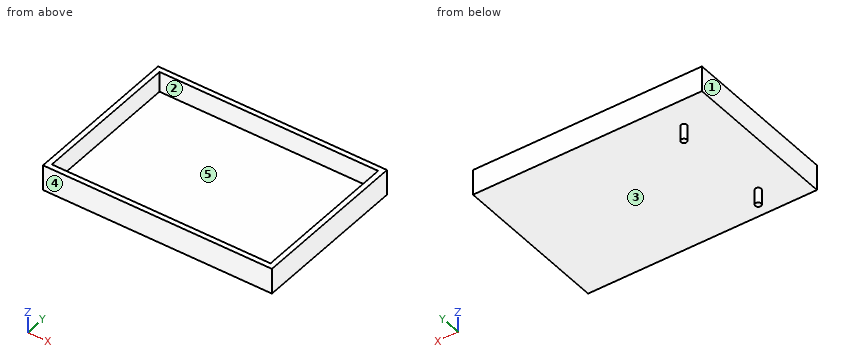
Autodesk Fusion 360 part; units mm, degrees
sketch "Sketch1" plane through (0, 0, 0) normal (0, 0, 1) x (1, 0, 0)
  line L0 (0, 0) -> (85.5, 0)
  line L1 (85.5, 0) -> (85.5, 58)
  line L2 (85.5, 58) -> (0, 58)
  line L3 (0, 58) -> (0, 0)
  line L4 (87.5, -2) -> (87.5, 60)
  line L5 (87.5, 60) -> (-2, 60)
  line L6 (-2, 60) -> (-2, -2)
  line L7 (-2, -2) -> (87.5, -2)
  dimension "d1" = 85.5
  dimension "d2" = 58
  dimension "d3" = 2
extrude "Extrude1" add sketch "Sketch1" along normal blind 10
sketch "Sketch2" plane through (0, 0, 0) normal (0, 0, 1) x (1, 0, 0)
  line L0 (0, 0) -> (85.5, 0)
  line L1 (85.5, 0) -> (85.5, 58)
  line L2 (85.5, 58) -> (0, 58)
  line L3 (0, 58) -> (0, 0)
  point P0 (85.5, 58)
extrude "Extrude2" add sketch "Sketch2" along normal blind 2
sketch "Sketch3" plane through (0, 0, 0) normal (0, 0, -1) x (1, 0, 0)
  line L0 (87.5, 2) -> (-2, 2)
  line L1 (-2, 2) -> (-2, -60)
  line L2 (-2, -60) -> (87.5, -60)
  line L3 (87.5, -60) -> (87.5, 2)
  line L4 (-2, -29) -> (87.5, -29)
  circle A0 centre (13, -9) radius 1.125
  circle A1 centre (13, -49) radius 1.125
  dimension "d8" = 2.25
  dimension "d9" = 2.25
  dimension "d10" = 20
  dimension "d11" = 20
  dimension "d14" = 15
extrude "Extrude3" add sketch "Sketch3" along normal blind 6 contours A0 | A1
sketch "Sketch4" plane through (0, 0, 0) normal (0, 0, -1) x (1, 0, 0)
  circle A0 centre (13, -9) radius 1.125
  circle A1 centre (13, -49) radius 1.125
  line L0 (87.5, 2) -> (-2, 2)
  line L1 (-2, 2) -> (-2, -60)
  line L2 (-2, -60) -> (87.5, -60)
  line L3 (87.5, -60) -> (87.5, 2)
For this review, take the finished solid that the model builds, in its own axes (mm). Face numbers are marked on the shaded views. A direction names the side the tool comes from. Round coordinates to 2 decimals unless told otherwise and drop trailing zeros. Order: outer loops, then holes, each group sorted by start corner. A loop starts at its lowest first (then second) coordinate and runs counter-clockwise, first axis right, second up.
Q1. We need section C-C, the plane y = 9. Give the boundary of the cut face in (x, z) (3 decimals).
Findings below:
outline: (-2, 0) - (11.875, 0) - (11.875, -6) - (14.125, -6) - (14.125, 0) - (87.5, 0) - (87.5, 10) - (85.5, 10) - (85.5, 2) - (0, 2) - (0, 10) - (-2, 10) - close
Q2. Machinability: for the marked faces 4 and 5, which of the approach directions +Z, -Z, +X, -X, +Y, -Y give a long, thin tool a straight path to every point of the face, cutting with its end or side? Answer none if there is none.
Findings below:
face 4: +Z, -Z, +X, -X, -Y
face 5: +Z
Q3. Wall thickness on line 1 (X direction, y = 29.5, z = 4.25); line 2 (Y direction, x = 2, z = 2.5); line 3 (Z direction, x = 67.5, y = 36.5): over which ranges is each line inside the solid? List them lowest first.
Findings below:
line 1: x = -2 to 0, 85.5 to 87.5
line 2: y = -2 to 0, 58 to 60
line 3: z = 0 to 2
Q4. Mouldability with a two-part tool opening along X and no side actions: class the marked faces 1, 2 and 3 as pulls with the +X half, pulls with the -X half, needs draft (parallel to the pull), parting line crosses it, or undercut.
Findings below:
face 1: pulls with the -X half
face 2: undercut
face 3: needs draft
Q5. We need section B-B, the plane x = 13. Give the boundary of the cut face in (y, z) (3 decimals), plus the area to 3 significant figures.
Findings below:
outline: (-2, 0) - (7.875, 0) - (7.875, -6) - (10.125, -6) - (10.125, 0) - (47.875, 0) - (47.875, -6) - (50.125, -6) - (50.125, 0) - (60, 0) - (60, 10) - (58, 10) - (58, 2) - (0, 2) - (0, 10) - (-2, 10) - close
area: 183 mm2
Q6. We need section D-D, the plane x = 50.5. Give the boundary of the cut face in (y, z).
Findings below:
outline: (-2, 0) - (60, 0) - (60, 10) - (58, 10) - (58, 2) - (0, 2) - (0, 10) - (-2, 10) - close
Q7. We need section A-A, the plane z = 8. Give the boundary of the cut face in (x, y), plus the area to 3 significant figures.
Findings below:
outline: (-2, -2) - (87.5, -2) - (87.5, 60) - (-2, 60) - close; hole (0, 0) - (85.5, 0) - (85.5, 58) - (0, 58) - close
area: 590 mm2
Q8. Insertion check: P1, Ø12, axis at x = 30, y = 11.5, coming from the -Z side; P2, Ø8, axis at x = 60, y = 18, coming from the +Z side. Each pin has a flat end and moves straight along its axis. Give the tip position at first contact, or say it passes through.
Findings below:
P1: stops at z = 0
P2: stops at z = 2
